```python
from build123d import *

# Parameters (mm, degrees)
SKETCH2_R           = 28.575
BOSS_EXTRUDE1_DEPTH = 92
SKETCH3_R           = 25.4
CUT_EXTRUDE1_DEPTH  = 110
SKETCH7_R           = 2.25
CUT_EXTRUDE2_DEPTH  = 110
CIRPATTERN1_COUNT   = 6
SKETCH8_R           = 2.25
CUT_EXTRUDE5_DEPTH  = 101.484134476
CIRPATTERN2_COUNT   = 6
CHAMFER1_SIZE       = 1


with BuildPart() as part:
    # Sketch2 → Boss-Extrude1 (new body)
    with BuildSketch(Plane(origin=(0, 0, 0), x_dir=(1, 0, 0), z_dir=(0, 1, 0))):
        with Locations(Location((0, 0, 0), (0, 0, 270))):
            Circle(SKETCH2_R)
    extrude(amount=-BOSS_EXTRUDE1_DEPTH)

    # Sketch3 → Cut-Extrude1 (cut)
    with BuildSketch(Plane(origin=(0, 0, 0), x_dir=(1, 0, 0), z_dir=(0, 1, 0))):
        with Locations(Location((0, 0, 0), (0, 0, 270))):
            Circle(SKETCH3_R)
    extrude(amount=-CUT_EXTRUDE1_DEPTH, mode=Mode.SUBTRACT)

    # Sketch7 → Cut-Extrude2 (cut)
    with BuildSketch(Plane(origin=(0, 0, 0), x_dir=(0, 0, -1), z_dir=(1, 0, 0))):
        with Locations((0, -5)):
            Circle(SKETCH7_R)
    cut_extrude2 = extrude(amount=-CUT_EXTRUDE2_DEPTH, mode=Mode.SUBTRACT)

    # CirPattern1: Cut-Extrude2 ×6 about axis
    cirpattern1_axis = Axis((0, 0, 0), (0, -1, 0))
    for i in range(1, CIRPATTERN1_COUNT):
        add(cut_extrude2.rotate(cirpattern1_axis, i * 360 / CIRPATTERN1_COUNT), mode=Mode.SUBTRACT)

    # Sketch8 → Cut-Extrude5 (cut, symmetric)
    with BuildSketch(Plane(origin=(0, 0, 0), x_dir=(0, 0, -1), z_dir=(1, 0, 0))):
        with Locations((0, -87)):
            Circle(SKETCH8_R)
    cut_extrude5 = extrude(amount=CUT_EXTRUDE5_DEPTH, both=True, mode=Mode.SUBTRACT)

    # CirPattern2: Cut-Extrude5 ×6 about axis
    cirpattern2_axis = Axis((0, 0, 0), (0, -1, 0))
    for i in range(1, CIRPATTERN2_COUNT):
        add(cut_extrude5.rotate(cirpattern2_axis, i * 360 / CIRPATTERN2_COUNT), mode=Mode.SUBTRACT)

    # Chamfer1
    chamfer1_edges = [part.edges().sort_by_distance(p)[0] for p in [
        (0, -92, -25.4),
        (0, 0, -25.4),
    ]]
    chamfer(chamfer1_edges, length=CHAMFER1_SIZE)


solid = part.part
```
Input: part model. Units: mm. Frame: model coordinates. Round coordinates to 2 decimals unless told otherwise and drop trailing zeros. Order: outer loops, then holes, each group sorted by start corner. A loop starts at its lowest first (then second) coordinate and runs counter-clockwise, first axis right, second up. Notation, with made-up numbers: (53.25, 21.5) - (68.25, 21.5) arc R28 ccw to (68.25, 44.5) - close; hole circle Ø8 at (57, 73). An arc over 180 degrees is marked (long way). One line per question, with ' | ' between items. Start each with the question number.
1) Pull-direction query (Z, two-part tool) for faces 1 (the flat face through (-25.3, -92, 8.3)), 2 (the cylindrical face through (-13.903, -89.196, 23.105)), 3 (the cylindrical face through (1.256, -45.356, -28.547)); classes: +Z half, -Z half, draft (parallel to the pull), parting line (faces both ways), or undercut.
2) Cut plane D-D, the plane y = -33. Return the cut outline in (x, z) (3 decimals).
3) Cut plane A-A, the plane x = 0. Return the cut outline in (y, z) (3 decimals).
4) Contact query for flat-ended pins moving along their axis: P1, Ø1, axis at x = 22, y = -60, coming from the -Z side; P2, Ø1.5, axis at y = -43, z = -14.5, coming from the +X side; P3, Ø4, axis at y = -14, z = 17.5, coming from the +X side. Output: stop coordinate, or through.
5) Cut plane C-C, the plane y = -87. Return the cut outline in (x, z) (3 decimals), then the cut area to 3 significant figures.
6) Cut plane B-B, the plane z = 0. Return the cut outline in (x, y) (3 decimals), then the cut area to 3 significant figures.
7) Ray query, probe 1 along Y at (x, z) = (26.5, 0); probe 2 along X at (y, z) = (-24, 0) (3 decimals); probe 3 along X at (y, z) = (-19, -23). Return the intervals inside material, ascending.
Worked out:
1) face 1: draft | face 2: undercut | face 3: parting line
2) outline: circle Ø57.15 at (0, 0); hole circle Ø50.8 at (0, 0)
3) outline: (-92, -28.575) - (0, -28.575) - (0, -26.4) - (-1, -25.4) - (-91, -25.4) - (-92, -26.4) - close; (-92, 26.4) - (-91, 25.4) - (-1, 25.4) - (0, 26.4) - (0, 28.575) - (-92, 28.575) - close
4) P1: stops at z = -18.82 | P2: stops at x = 25.05 | P3: stops at x = 24.01
5) outline: (-28.486, -2.25) arc R28.575 ccw to (-16.192, -23.545) - (-14.599, -20.786) arc R25.4 cw to (-25.3, -2.25) - close; (-28.486, 2.25) - (-25.3, 2.25) arc R25.4 cw to (-14.599, 20.786) - (-16.192, 23.545) arc R28.575 ccw to start; (-12.295, -25.795) arc R28.575 ccw to (12.295, -25.795) - (10.702, -23.036) arc R25.4 cw to (-10.702, -23.036) - close; (-12.295, 25.795) - (-10.702, 23.036) arc R25.4 cw to (10.702, 23.036) - (12.295, 25.795) arc R28.575 ccw to start; (14.599, -20.786) - (16.192, -23.545) arc R28.575 ccw to (28.486, -2.25) - (25.3, -2.25) arc R25.4 cw to start; (14.599, 20.786) arc R25.4 cw to (25.3, 2.25) - (28.486, 2.25) arc R28.575 ccw to (16.192, 23.545) - close | area: 453 mm^2
6) outline: (-28.575, -92) - (-26.4, -92) - (-25.4, -91) - (-25.4, -89.25) - (-28.575, -89.25) - close; (-28.575, -84.75) - (-25.4, -84.75) - (-25.4, -7.25) - (-28.575, -7.25) - close; (-28.575, -2.75) - (-25.4, -2.75) - (-25.4, -1) - (-26.4, 0) - (-28.575, 0) - close; (25.4, -91) - (26.4, -92) - (28.575, -92) - (28.575, -89.25) - (25.4, -89.25) - close; (25.4, -84.75) - (28.575, -84.75) - (28.575, -7.25) - (25.4, -7.25) - close; (25.4, -2.75) - (28.575, -2.75) - (28.575, 0) - (26.4, 0) - (25.4, -1) - close | area: 525 mm^2
7) probe 1: y = -92 to -89.25, -84.75 to -7.25, -2.75 to 0 | probe 2: x = -28.575 to -25.4, 25.4 to 28.575 | probe 3: x = -16.96 to -10.78, 10.78 to 16.96
